Input: part model. Units: mm. Frame: model coordinates. Face numbers are marked on the shaded views. Give positions to 0.01 mm unless a question says otherwise; leave off trailing zeros. Loops run counter-clockwise (first coordinate to the right, second up) from the corner with the lowest first, then second, coordinate; pieces in that order, holes last. Notation, with made-up numbers: (-10, 82.25) - (43, 82.25) arc R31 cw to (43, 115.25) - close; hole circle Ø7 at (13.5, 9.5). An arc over 180 degrees is marked (long way). Answer as a JSON object with one key per item and string values.
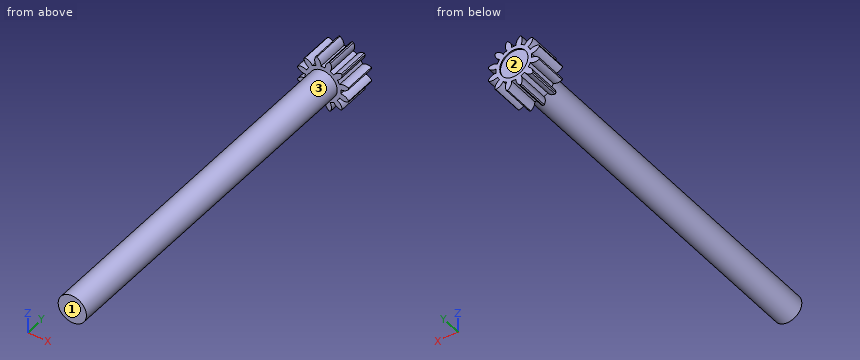
from build123d import *

# Parameters (mm, degrees)
BOSS_EXTRUDE1_DEPTH = 7
SKETCH2_R           = 3
CUT_EXTRUDE1_DEPTH  = 7
BOSS_EXTRUDE2_START = -0.25
SKETCH2_2_R         = 3
BOSS_EXTRUDE2_DEPTH = 82.81


with BuildPart() as part:
    # Sketch1 → Boss-Extrude1 (new body)
    with BuildSketch(Plane(origin=(0, 0, 0), x_dir=(1, 0, 0), z_dir=(0, 1, 0))):
        with BuildLine():
            ThreePointArc((-4.057364733, 3.859765721), (-3.757286187, 2.934610179), (-3.042339168, 2.275208427))
            ThreePointArc((-3.042339168, 2.275208427), (-3.290030509, 1.8995), (-3.491557881, 1.497138792))
            ThreePointArc((-3.491557881, 1.497138792), (-4.420090059, 1.786600197), (-5.371337534, 1.583898071))
            ThreePointArc((-5.371337534, 1.583898071), (-5.409184627, 1.449386653), (-5.443663792, 1.313972801))
            ThreePointArc((-5.443663792, 1.313972801), (-4.721210377, 0.662803872), (-3.77234722, 0.449218713))
            ThreePointArc((-3.77234722, 0.449218713), (-3.799, 0), (-3.77234722, -0.449218713))
            ThreePointArc((-3.77234722, -0.449218713), (-4.721210377, -0.662803872), (-5.443663792, -1.313972801))
            ThreePointArc((-5.443663792, -1.313972801), (-5.409184627, -1.449386653), (-5.371337534, -1.583898071))
            ThreePointArc((-5.371337534, -1.583898071), (-4.420090059, -1.786600197), (-3.491557881, -1.497138792))
            ThreePointArc((-3.491557881, -1.497138792), (-3.290030509, -1.8995), (-3.042339168, -2.275208427))
            ThreePointArc((-3.042339168, -2.275208427), (-3.757286187, -2.934610179), (-4.057364733, -3.859765721))
            ThreePointArc((-4.057364733, -3.859765721), (-3.959797975, -3.959797975), (-3.859765721, -4.057364733))
            ThreePointArc((-3.859765721, -4.057364733), (-2.934610179, -3.757286187), (-2.275208427, -3.042339168))
            ThreePointArc((-2.275208427, -3.042339168), (-1.8995, -3.290030509), (-1.497138792, -3.491557881))
            ThreePointArc((-1.497138792, -3.491557881), (-1.786600197, -4.420090059), (-1.583898071, -5.371337534))
            ThreePointArc((-1.583898071, -5.371337534), (-1.449386653, -5.409184627), (-1.313972801, -5.443663792))
            ThreePointArc((-1.313972801, -5.443663792), (-0.662803872, -4.721210377), (-0.449218713, -3.77234722))
            ThreePointArc((-0.449218713, -3.77234722), (0, -3.799), (0.449218713, -3.77234722))
            ThreePointArc((0.449218713, -3.77234722), (0.662803872, -4.721210377), (1.313972801, -5.443663792))
            ThreePointArc((1.313972801, -5.443663792), (1.449386653, -5.409184627), (1.583898071, -5.371337534))
            ThreePointArc((1.583898071, -5.371337534), (1.786600197, -4.420090059), (1.497138792, -3.491557881))
            ThreePointArc((1.497138792, -3.491557881), (1.8995, -3.290030509), (2.275208427, -3.042339168))
            ThreePointArc((2.275208427, -3.042339168), (2.934610179, -3.757286187), (3.859765721, -4.057364733))
            ThreePointArc((3.859765721, -4.057364733), (3.959797975, -3.959797975), (4.057364733, -3.859765721))
            ThreePointArc((4.057364733, -3.859765721), (3.757286187, -2.934610179), (3.042339168, -2.275208427))
            ThreePointArc((3.042339168, -2.275208427), (3.290030509, -1.8995), (3.491557881, -1.497138792))
            ThreePointArc((3.491557881, -1.497138792), (4.420090059, -1.786600197), (5.371337534, -1.583898071))
            ThreePointArc((5.371337534, -1.583898071), (5.409184627, -1.449386653), (5.443663792, -1.313972801))
            ThreePointArc((5.443663792, -1.313972801), (4.721210377, -0.662803872), (3.77234722, -0.449218713))
            ThreePointArc((3.77234722, -0.449218713), (3.799, 0), (3.77234722, 0.449218713))
            ThreePointArc((3.77234722, 0.449218713), (4.721210377, 0.662803872), (5.443663792, 1.313972801))
            ThreePointArc((5.443663792, 1.313972801), (5.409184627, 1.449386653), (5.371337534, 1.583898071))
            ThreePointArc((5.371337534, 1.583898071), (4.420090059, 1.786600197), (3.491557881, 1.497138792))
            ThreePointArc((3.491557881, 1.497138792), (3.290030509, 1.8995), (3.042339168, 2.275208427))
            ThreePointArc((3.042339168, 2.275208427), (3.757286187, 2.934610179), (4.057364733, 3.859765721))
            ThreePointArc((4.057364733, 3.859765721), (3.959797975, 3.959797975), (3.859765721, 4.057364733))
            ThreePointArc((3.859765721, 4.057364733), (2.934610179, 3.757286187), (2.275208427, 3.042339168))
            ThreePointArc((2.275208427, 3.042339168), (1.8995, 3.290030509), (1.497138792, 3.491557881))
            ThreePointArc((1.497138792, 3.491557881), (1.786600197, 4.420090059), (1.583898071, 5.371337534))
            ThreePointArc((1.583898071, 5.371337534), (1.449386653, 5.409184627), (1.313972801, 5.443663792))
            ThreePointArc((1.313972801, 5.443663792), (0.662803872, 4.721210377), (0.449218713, 3.77234722))
            ThreePointArc((0.449218713, 3.77234722), (0, 3.799), (-0.449218713, 3.77234722))
            ThreePointArc((-0.449218713, 3.77234722), (-0.662803872, 4.721210377), (-1.313972801, 5.443663792))
            ThreePointArc((-1.313972801, 5.443663792), (-1.449386653, 5.409184627), (-1.583898071, 5.371337534))
            ThreePointArc((-1.583898071, 5.371337534), (-1.786600197, 4.420090059), (-1.497138792, 3.491557881))
            ThreePointArc((-1.497138792, 3.491557881), (-1.8995, 3.290030509), (-2.275208427, 3.042339168))
            ThreePointArc((-2.275208427, 3.042339168), (-2.934610179, 3.757286187), (-3.859765721, 4.057364733))
            ThreePointArc((-3.859765721, 4.057364733), (-3.959797975, 3.959797975), (-4.057364733, 3.859765721))
        make_face()
    extrude(amount=BOSS_EXTRUDE1_DEPTH)

    # Sketch2 → Cut-Extrude1 (cut)
    with BuildSketch(Plane(origin=(0, 7, 0), x_dir=(1, 0, 0), z_dir=(0, 1, 0))):
        Circle(SKETCH2_R)
    extrude(amount=-CUT_EXTRUDE1_DEPTH, mode=Mode.SUBTRACT)

    # Sketch2<2> → Boss-Extrude2 (add)
    with BuildSketch(Plane(origin=(0, 7, 0), x_dir=(1, 0, 0), z_dir=(0, 1, 0)).offset(BOSS_EXTRUDE2_START)):
        Circle(SKETCH2_2_R)
    extrude(amount=-BOSS_EXTRUDE2_DEPTH)


solid = part.part
Item 1: Cut plane A-A (y = -27). Return loops of the section in (x, z), then the cut area to 3 significant figures.
Geometry check:
{"outline": "circle Ø6 at (0, 0)", "area": "28.3 mm2"}
Item 2: Material intervals for line 1 (Y direction, x = -0.5, z = -1.5); line 2 (Y direction, x = -2.5, z = -3); line 3 (X direction, y = -49.5, z = 0.25), sorted ascending. Write a range as [from, to].
Geometry check:
{"line 1": "y = [-76.06, 6.75]", "line 2": "y = [0, 7]", "line 3": "x = [-2.99, 2.99]"}
Item 3: Mould query, pull axis X, two halves, no side actions, for the marked faces 1, 2 and 3. Classes: released by +X, released by -X, zero draft, split by the parting line, or undercut.
Geometry check:
{"face 1": "zero draft", "face 2": "undercut", "face 3": "split by the parting line"}
Item 4: Contact query for flat-ended pins moving along their axis: P1, Ø2, axis at y = -40, z = 1.5, coming from the -X side; P2, Ø5, axis at y = -40, z = -4, coming from the -X side; P3, Ø3, axis at y = -25, z = 3.5, coming from the +X side. Output: stop coordinate, or through.
Geometry check:
{"P1": "stops at x = -2.96", "P2": "stops at x = -2.6", "P3": "stops at x = 2.24"}
